For this review, use the dimensioned drawing (mm, ordinates from the lowest corner) and the shaded views. A direction names the side the tool comes from. Give positions to 0.01 mm unless a question says otherwise; leave off trailing zeros. Loops run counter-clockwise (first coordinate to the right, second up) from the corner with the lowest first, then second, coordinate; pieces in that order, holes last. Notation, with made-up numbers: (-19.75, 26) -> (-10.75, 26) arc R34 cw to (-10.75, 65) -> close; hole circle Ø10 at (-16.5, 32.5). An arc over 180 degrees is marked (long way). Write each question's results on one line, items separated by ' | '. Start each with the question number.
Q1. Insertion check: pin 1 Ø3 at (x, y) = (1.5, 6) entering from +Z; pin 2 Ø1.3 at (y, z) = (5, 26.5) entering from -X; pin 3 Ø2 at (x, z) = (2.68, 25.505) entering from +Y; pin 4 Ø3 at (y, z) = (5.5, 27.5) entering from +X. Each pin has a flat end and moves straight along its axis. Give the tip position at first contact, or say it passes through.
Q2. Machinability: for the marked faces 1 and 2, which of the approach directions +Z, -Z, +X, -X, +Y, -Y give a long, thin tool a straight path to every point of the face, cutting with its end or side? Answer none if there is none.
Q3. Wall thickness on L1, parallel to Z at x = 2.68, y = 0.95; L2, parallel to X at y = 6.5, z = 27; L3, parallel to X at y = 2.25, z = 24.5: over which ranges is each line inside the solid? List them lowest first. Write a range as [from, to].
Q4. We need section A-A (y = 5). Write out the cut boundary in (x, z) (3 decimals), plus the area to 3 significant figures.
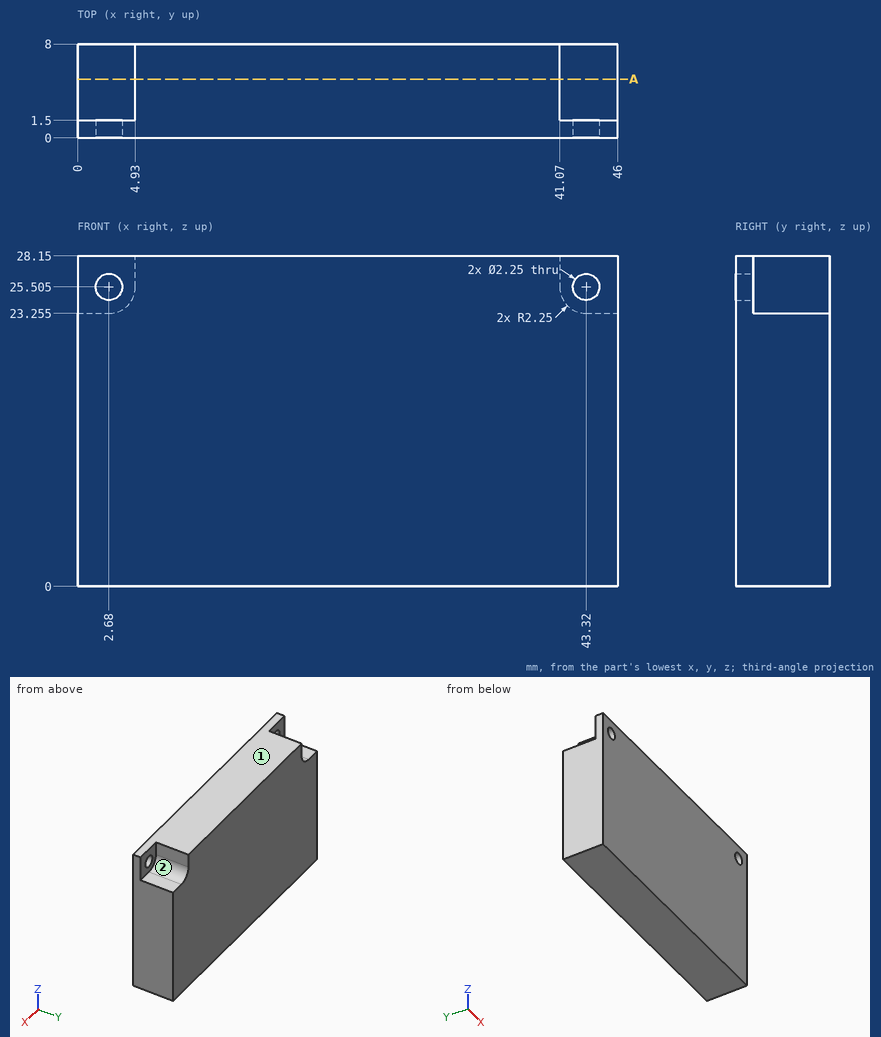
Output:
1) pin 1: z = 23.28 | pin 2: x = 4.93 | pin 3: through | pin 4: x = 41.07
2) face 1: +Z, +X, -X, +Y, -Y | face 2: +Z, +X, +Y
3) L1: [0, 24.38], [26.63, 28.15] | L2: [4.93, 41.07] | L3: [4.69, 41.31]
4) outline: (0, 0) -> (46, 0) -> (46, 23.255) -> (43.32, 23.255) arc R2.25 cw to (41.07, 25.505) -> (41.07, 28.15) -> (4.93, 28.15) -> (4.93, 25.505) arc R2.25 cw to (2.68, 23.255) -> (0, 23.255) -> close | area: 1,250 mm2
